Part print with two shaded views. Sizes in mm from the minimum x, y, z corner. A direction names the side the tool comes from. Give positions to 0.01 mm unless a question says otherwise; leave off trailing zeros. Write each loop counter-clockwise with the first axis right and the second up, starting at its lowest first coordinate (ties: lowest second). Pieces come first, ordered by that corner, then holes. Notation, with made-up numbers: (25.5, 9.25) -> (38.5, 9.25) arc R33 ccw to (38.5, 43.25) -> close; hole circle Ø7 at (38, -30.75). An arc over 180 degrees is marked (long way). Answer as a JSON object with one key per item and string values.
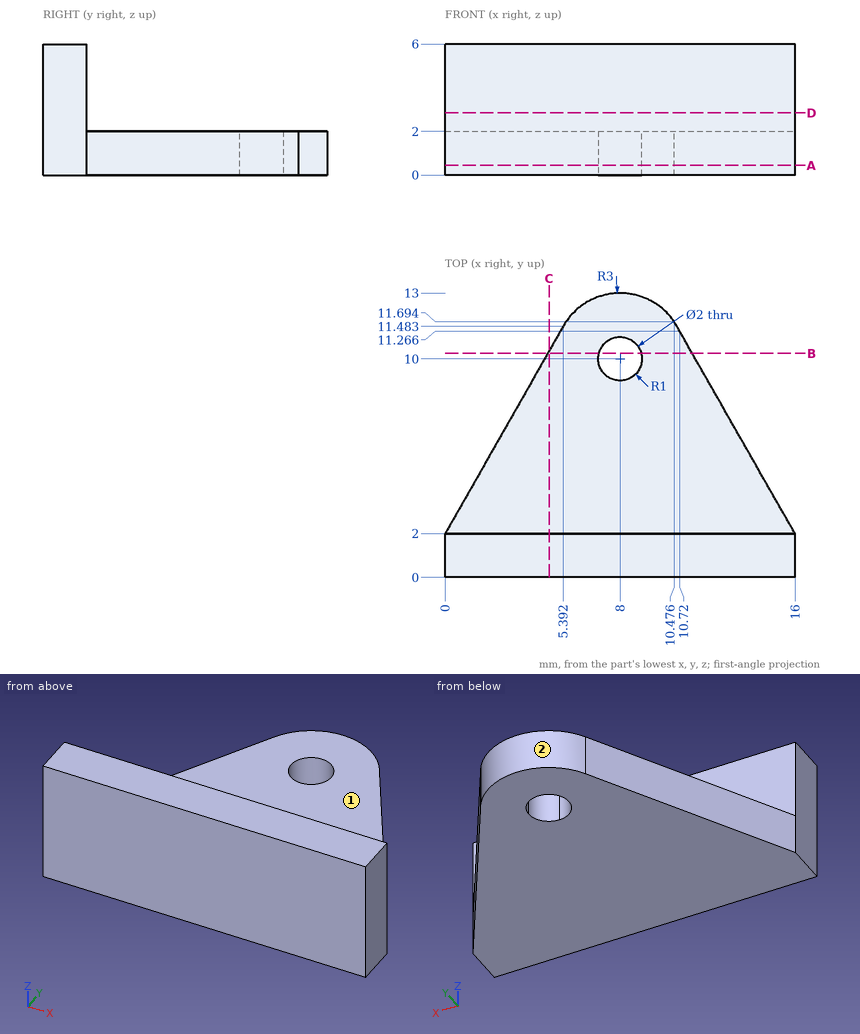
1) Slice it at B-B (y = 10.25). List the corners of the cut face in (x, z).
Model answer:
{"outline": "(4.69, 0) -> (7.03, 0) -> (7.03, 2) -> (4.69, 2) -> close; (8.97, 0) -> (11.3, 0) -> (11.3, 2) -> (8.97, 2) -> close"}
2) Wall check: probe 1 along Z at (x, y) = (9.5, 8); probe 2 along X at (y, z) = (10, 0.75). Give the ranges that are in metal, low to high.
Model answer:
{"probe 1": "z = 0 to 2", "probe 2": "x = 4.55 to 7, 9 to 11.44"}
3) Pin check, flat tips, straight feed: pin 1 (3.5 mm diameter, centred on x = 10.5, y = 9, fed in from +Z); pin 2 (3 mm diameter, centred on y = 4, z = 1.5, fed in from -X) (1 decimal); pin 3 (2 mm diameter, centred on x = 12, z = 5, fed in from +Y). Stop position of each tip, or through.
Model answer:
{"pin 1": "stops at z = 2", "pin 2": "stops at x = 0.3", "pin 3": "stops at y = 2"}
4) 3-axis set-ups, long thin cutter, end or side, ignore diameter. For the marked faces 1 and 2: which of +Z, -Z, +X, -X, +Y, -Y reach the whole face in a straight line?
Model answer:
{"face 1": "+Z, +X, -X, +Y", "face 2": "+Z, -Z, +Y"}
5) Slice it at D-D (z = 2.85). List the corners of the cut face in (x, y).
Model answer:
{"outline": "(0, 0) -> (16, 0) -> (16, 2) -> (0, 2) -> close"}
6) Slice it at C-C (x = 4.75). List the corners of the cut face in (y, z).
Model answer:
{"outline": "(0, 0) -> (10.35, 0) -> (10.35, 2) -> (2, 2) -> (2, 6) -> (0, 6) -> close"}
7) Slice it at A-A (z = 0.45). List the corners of the cut face in (x, y) (1 decimal).
Model answer:
{"outline": "(0, 0) -> (16, 0) -> (16, 2) -> (10.5, 11.7) arc R3 ccw to (5.4, 11.5) -> (0, 2) -> close; hole circle Ø2 at (8, 10)"}
